Part model, mm, in its own coordinate system. Give positions to 0.01 mm unless a question says otherwise; leave off trailing zeros. Write each loop counter-clockwise with the first axis right and the second up, starting at its lowest first coordinate (ties: lowest second). Pieces come first, ordered by that corner, then holes. Notation, with made-up numbers: M 15,78.5 L 56,78.5 A28 cw 56,114.5 Z; hole C -35.5,-11.5 d10. An arc over 180 degrees is marked long. Answer as CSV lines item,"result". Start each with the question number.
1) Slice it at A-A, the plane x = -15.25. Give the cut face in (y, z).
2) Slice it at B-B, the plane z = -0.95. Give the cut face in (x, y) (3 decimals), plus the area to 3 significant figures.
3) Pin check, flat tip, straight feed: pin 1 Ø10 at (x, y) = (-7, -4) entering from -Z. Stop position of the tip, or through.
4) Wall check: line 1 along Y through (x, z) = (-8.75, -0.75); line 2 along Y through (x, z) = (-9, 0.9); line 3 along X through (y, z) = (-5.5, -0.6). Give the ranges that are in metal, low to high. Write a range as from..to.
5) Slice it at C-C, the plane y = -30.5. Give the cut face in (x, z), plus the area to 3 significant figures.
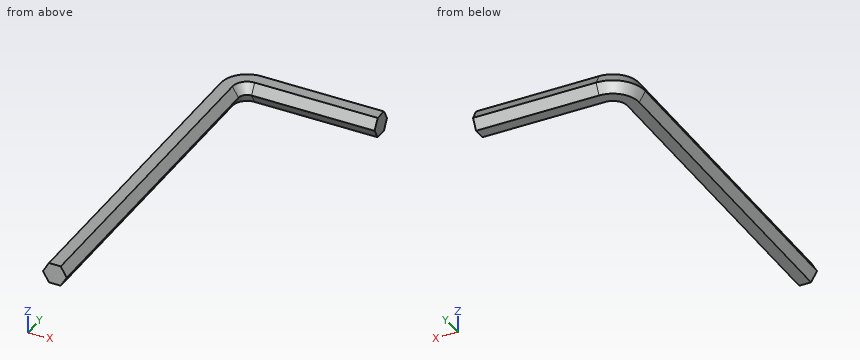
```python
from build123d import *

# Parameters (mm, degrees)
BOSS_EXTRUDE1_DEPTH = 19.05
REVOLVE4_ANGLE      = 90
BOSS_EXTRUDE2_DEPTH = 50.8


with BuildPart() as part:
    # Sketch1 → Boss-Extrude1 (new body)
    with BuildSketch(Plane(origin=(0, 0, 0), x_dir=(0, 0, -1), z_dir=(1, 0, 0))):
        Polygon((1.5875, 0.916543552), (0, 1.833087105), (-1.5875, 0.916543552), (-1.5875, -0.916543552), (0, -1.833087105), (1.5875, -0.916543552), align=None)
    extrude(amount=-BOSS_EXTRUDE1_DEPTH)

    # Sketch3 → Revolve4 (revolve)
    with BuildSketch(Plane.ZY.offset(19.05)):
        Polygon((-1.5875, 0.916543552), (-1.5875, -0.916543552), (0, -1.833087105), (1.5875, -0.916543552), (1.5875, 0.916543552), (0, 1.833087105), align=None)
    revolve(axis=Axis((-19.05, -3.175, 0), (0, 0, 1)), revolution_arc=REVOLVE4_ANGLE)

    # Sketch4 → Boss-Extrude2 (add)
    with BuildSketch(Plane.XZ.offset(3.175)):
        Polygon((-24.058087105, 0), (-23.141543552, -1.5875), (-21.308456448, -1.5875), (-20.391912895, 0), (-21.308456448, 1.5875), (-23.141543552, 1.5875), align=None)
    extrude(amount=BOSS_EXTRUDE2_DEPTH)


solid = part.part
```
Found:
1,outline,"M -1.83,0 L -0.92,-1.59 L 0.92,-1.59 L 1.83,0 L 0.92,1.59 L -0.92,1.59 Z"
2,outline,"M -23.51,-53.975 L -20.94,-53.975 L -20.94,-3.175 A1.89 cw -19.05,-1.285 L 0,-1.285 L 0,1.285 L -19.05,1.285 A4.46 ccw -23.51,-3.175 Z"
2,area,"192 mm²"
3,pin 1,"z = -1.59"
4,line 1,"-1.4..1.4"
4,line 2,"-1.31..1.31"
4,line 3,"-23.71..-20.74"
5,outline,"M -24.06,0 L -23.14,-1.59 L -21.31,-1.59 L -20.39,0 L -21.31,1.59 L -23.14,1.59 Z"
5,area,"8.73 mm²"
